Verification items for the finished model (mm, model axes). Face numbers are marked on the shaded views. Give positions to 0.01 mm unless a question says otherwise; leave off trailing zeros. Loops run counter-clockwise (first coordinate to the right, second up) from the corner with the lowest first, then second, coordinate; pieces in that order, holes last. Notation, with made-up numbers: (72.5, 29) - (80.5, 29) arc R24 ccw to (80.5, 66) - close; hole circle Ø10 at (-25, 23.5). An arc over 180 degrees is marked (long way). Answer in a Markdown table with one row per item.
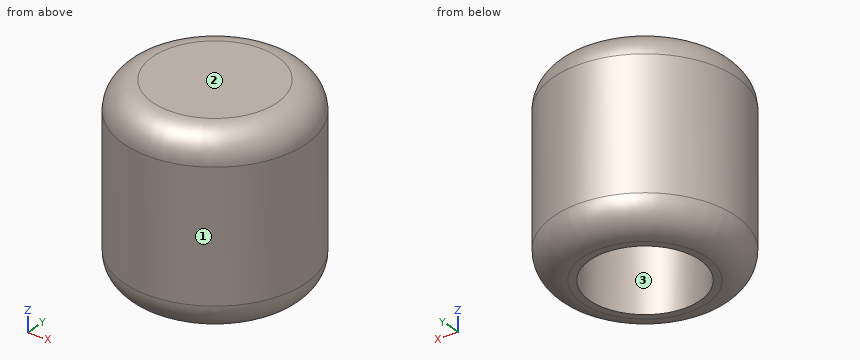
```python
from build123d import *

# Parameters (mm, degrees)
F0_R     = 8.0375
F0_R_2   = 4.8625
F1_DEPTH = 6.35
F2_R     = 8.0375
F3_DEPTH = 10.16
F4_R     = 2.54
F5_R     = 4.4
F6_DEPTH = 6.35
F7_R     = 2.54


with BuildPart() as f1:
    # F0 (on Top) → F1 (new body)
    with BuildSketch(Plane.XY):
        Circle(F0_R)
        Circle(F0_R_2, mode=Mode.SUBTRACT)
    extrude(amount=F1_DEPTH)

    # F2 (on face) → F3 (join)
    with BuildSketch(Plane.XY.offset(6.35)):
        Circle(F2_R)
    extrude(amount=F3_DEPTH)

    # F4
    f4_edges = [f1.edges().sort_by_distance(p)[0] for p in [
        (-8.0375, 0, 0),
    ]]
    fillet(f4_edges, radius=F4_R)

    # F5 (on face) → F6 (cut)
    with BuildSketch(Plane(origin=(0, 0, 6.35), x_dir=(1, 0, 0), z_dir=(0, 0, -1))):
        Circle(F5_R)
    extrude(amount=-F6_DEPTH, mode=Mode.SUBTRACT)

    # F7
    f7_edges = [f1.edges().sort_by_distance(p)[0] for p in [
        (-8.0375, 0, 16.51),
    ]]
    fillet(f7_edges, radius=F7_R)


solid = f1.part
```
Q1. Draft check along X on the marked faces 1, 2 and 3. Enter one of: +X half, -X half, draft (parallel to the pull), parting line (faces both ways), or undercut.
Completed:
| item | result |
|---|---|
| face 1 | parting line |
| face 2 | draft |
| face 3 | undercut |
Q2. Thickness scan on line 1 (Y direction, x = 0, z = 11); line 2 (Y direction, x = -0.5, z = 2.5); line 3 (X direction, y = -0.5, z = 12.5). Record the ranges inside material, lowest first.
Completed:
| item | result |
|---|---|
| line 1 | -8.04 to -4.4, 4.4 to 8.04 |
| line 2 | -8.02 to -4.84, 4.84 to 8.02 |
| line 3 | -8.02 to -4.37, 4.37 to 8.02 |
Q3. Sectioned sample at D-D (z = 4.5). Record the cut outline in (x, y) (1 decimal).
Completed:
| item | result |
|---|---|
| outline | circle Ø16.1 at (0, 0); hole circle Ø9.7 at (0, 0) |
Q4. Sectioned sample at C-C (z = 9). Record the cut outline in (x, y) (1 decimal).
Completed:
| item | result |
|---|---|
| outline | circle Ø16.1 at (0, 0); hole circle Ø8.8 at (0, 0) |
Q5. Go/stop test with flat-tipped pins: P1, Ø9.5, axis at x = -1, y = -1, coming from the -Z side; P2, Ø5, axis at x = 1.5, y = 0, coming from the -Z side; P3, Ø4, axis at y = 5.5, z = 10, coming from the -X side; P4, Ø4, axis at x = -3, z = 3.5, coming from the -Y side. Record where each tip stops, or that it passes through.
Completed:
| item | result |
|---|---|
| P1 | z = 0 |
| P2 | z = 12.7 |
| P3 | x = -7.24 |
| P4 | y = -7.98 |
Q6. Sectioned sample at A-A (y = 0). Record the cut outline in (x, z).
Completed:
| item | result |
|---|---|
| outline | (-8.04, 2.54) arc R2.54 ccw to (-5.5, 0) - (-4.86, 0) - (-4.86, 6.35) - (-4.4, 6.35) - (-4.4, 12.7) - (4.4, 12.7) - (4.4, 6.35) - (4.86, 6.35) - (4.86, 0) - (5.5, 0) arc R2.54 ccw to (8.04, 2.54) - (8.04, 13.97) arc R2.54 ccw to (5.5, 16.51) - (-5.5, 16.51) arc R2.54 ccw to (-8.04, 13.97) - close |
